Geometry: see drawing. Coordinates: mm, zero at the bounding-box minimum. A direction names the side the tool comes from. Coordinates: 2 decimals unless noted, no trailing zeros. Loops run counter-clockwise (first coordinate to the right, second up) from the corner with the lowest first, then second, coordinate; pieces in that order, holes last. Notation, with made-up numbers: (44.25, -15.5) - (94.25, -15.5) arc R17 cw to (94.25, 2.5) - close; hole circle Ø2 at (-13.5, -36). An arc over 180 degrees is marked (long way). Use one line per item in the form item = value.
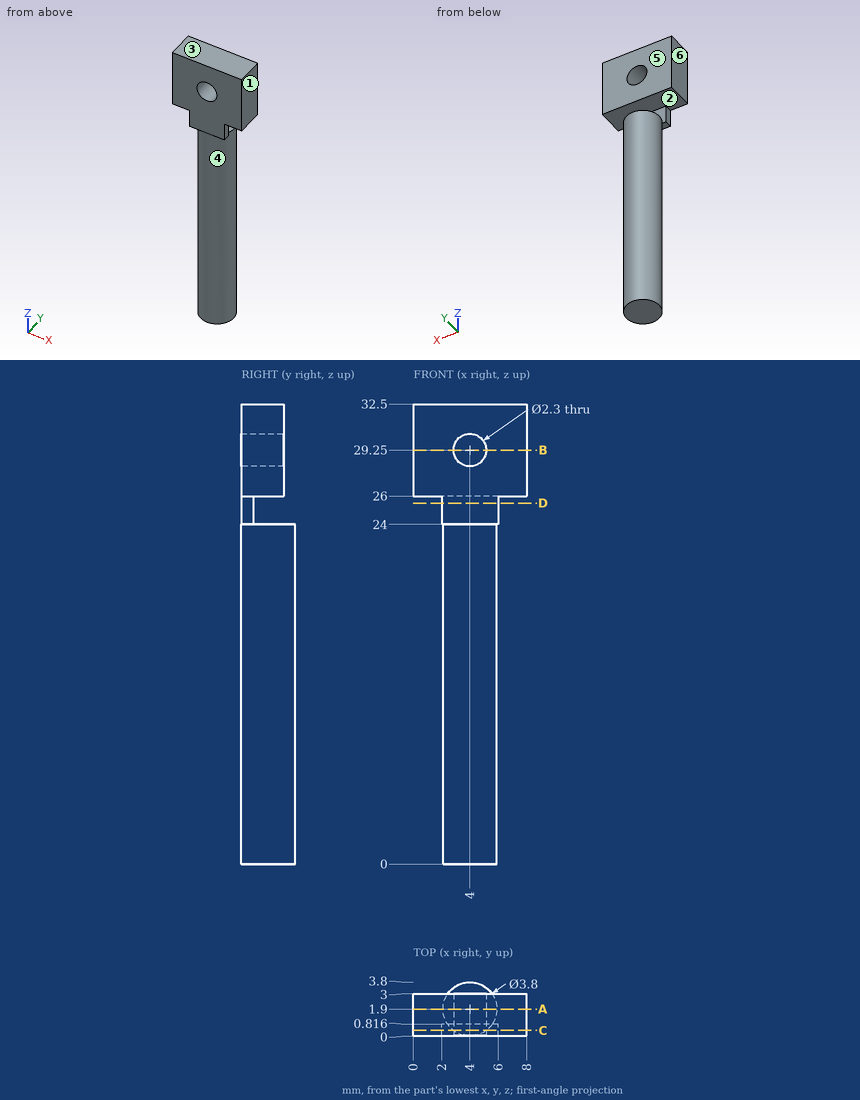
Q1. First-contact query: P1, Ø0.9, axis at x = 3, y = 0.5, coming from the -Z side; P2, Ø0.7, axis at y = 0, z = 25, coming from the +X side; P3, Ø1.5, axis at y = 1, z = 13.5, coming from the +X side; P4, Ø3, axis at x = 6.5, z = 10.5, coming from the +Y side. Flat tips, straight axial feed; report the tip coordinate or a pass-through.
Check values:
P1 = 0
P2 = 6
P3 = 5.89
P4 = 3.52
Q2. Ray query, line 1 along X through (y, z) = (0.7, 29.25); line 2 along Z through (x, y) = (5.75, 1.85); line 3 along Z through (x, y) = (4, 3.5). Return the intervals inside material, ascending. Write a range as [from, to].
Check values:
line_1 = [0, 2.85], [5.15, 8]
line_2 = [0, 24], [26, 32.5]
line_3 = [0, 24]
Q3. Set-up query: the marked faces 4, 5 and 6. Return all of +Z, -Z, +X, -X, +Y, -Y with unobstructed straight access to the full face (end or side cutting, diameter ignored); none if empty.
Check values:
face_4 = -Z
face_5 = +Z, +X, -X, +Y
face_6 = +Z, -Z, -X, +Y, -Y
Q4. Cut plane D-D, the plane z = 25.5. Return loops of the section in (x, y).
Check values:
outline = (2, 0) - (6, 0) - (6, 0.82) - (2, 0.82) - close
Q5. Cut plane A-A, the plane y = 1.9. Return loops of the section in (x, z), then the cut area to 3 significant figures.
Check values:
outline = (0, 26) - (8, 26) - (8, 32.5) - (0, 32.5) - close; (2.1, 0) - (5.9, 0) - (5.9, 24) - (2.1, 24) - close; hole circle Ø2.3 at (4, 29.25)
area = 139 mm²
Q6. Cut plane C-C, the plane y = 0.4. Return loops of the section in (x, z), then the cut area to 3 significant figures.
Check values:
outline = (0, 26) - (2, 26) - (2, 24) - (2.83, 24) - (2.83, 0) - (5.17, 0) - (5.17, 24) - (6, 24) - (6, 26) - (8, 26) - (8, 32.5) - (0, 32.5) - close; hole circle Ø2.3 at (4, 29.25)
area = 112 mm²
Q7. Cut plane B-B, the plane z = 29.25. Return loops of the section in (x, y).
Check values:
outline = (0, 0) - (2.85, 0) - (2.85, 3) - (0, 3) - close; (5.15, 0) - (8, 0) - (8, 3) - (5.15, 3) - close
Q8. Pull-direction query (Z, two-part tool) for the marked faces 1, 2 and 3; classes: pulls with the +Z half, pulls with the -Z half, needs draft (parallel to the pull), parting line crosses it, or undercut.
Check values:
face_1 = needs draft
face_2 = undercut
face_3 = pulls with the +Z half
